Build history of the part. All positions in model axes, mm. Face numbers are marked on the shaded views. A direction names the side the tool comes from. Give positions to 0.01 mm unless a question says otherwise; leave off trailing zeros. Loops run counter-clockwise (first coordinate to the right, second up) from the corner with the lowest first, then second, coordinate; pieces in that order, holes last.
1) Band-saw the part on A-A on z = 4.25. List the corners of the cut face in (x, y), then the cut area to 3 significant figures.
2) Band-saw the part on B-B on y = 15. List the corners of the cut face in (x, z).
3) 3-axis set-ups, long thin cutter, end or side, ignore diameter. For the marked faces 1, 2, 3, 4 and 5: which of +Z, -Z, +X, -X, +Y, -Y reach the whole face in a straight line?
4) Band-saw the part on C-C on x = 18. List the corners of the cut face in (y, z).
5) Wall check: line 1 (X direction, y = 13, z = 7); line 2 (X direction, y = 19.5, z = 3.25); line 3 (Y direction, x = 0.5, z = 9.75). Give the ranges that are in metal, low to high.
6) Two-plate mould, pull along X, no slides. Class the marked faces 6, 7 and 8: +X half, -X half, draft (parallel to the pull), parting line (faces both ways), or undercut.
7) Band-saw the part on D-D on y = 0. List the corners of the cut face in (x, z), then the cut area to 3 significant figures.
8) Flat gauge pins, fed straight in: P1, Ø5.5, axis at y = 21, z = 7.5, coming from the +X side; P2, Ø5, axis at x = 1, z = 3, coming from the +Y side; P3, Ø3, axis at x = 69.5, z = 6.5, coming from the +Y side. Where does each tip first touch, or does it go through?
```python
from build123d import *

# Parameters (mm, degrees)
SKETCH1_R           = 2.5
BOSS_EXTRUDE1_DEPTH = 10


with BuildPart() as part:
    # Sketch1 → Boss-Extrude1 (new body)
    with BuildSketch(Plane.XY):
        with BuildLine():
            Line((-11.526582654, 6), (20.973417346, 6))
            ThreePointArc((20.973417346, 6), (28.044485158, 8.928932188), (30.973417346, 16))
            Line((30.973417346, 16), (30.973417346, 41.837168574))
            ThreePointArc((30.973417346, 41.837168574), (32.455779256, 43.769020227), (34.705468153, 42.837168574))
            Line((34.705468153, 42.837168574), (55.973417346, 6))
            Line((55.973417346, 6), (67.348943548, 12.567663115))
            Line((67.348943548, 12.567663115), (64.080994355, 18.227917153))
            ThreePointArc((64.080994355, 18.227917153), (64.080994355, 20.227917153), (65.813045163, 21.227917153))
            Line((65.813045163, 21.227917153), (72.163898124, 21.227917153))
            ThreePointArc((72.163898124, 21.227917153), (75.663898124, 20.290094979), (78.22607595, 17.727917153))
            Line((78.22607595, 17.727917153), (78.411121374, 17.407409077))
            ThreePointArc((78.411121374, 17.407409077), (79.110424332, 15.719142393), (79.348943548, 13.907409077))
            Line((79.348943548, 13.907409077), (79.348943548, 9.680911769))
            ThreePointArc((79.348943548, 9.680911769), (78.411121374, 6.180911769), (75.848943548, 3.618733942))
            Line((75.848943548, 3.618733942), (60.813163308, -5.062177826))
            ThreePointArc((60.813163308, -5.062177826), (59.124896624, -5.761480784), (57.313163308, -6))
            Line((57.313163308, -6), (-11.526582654, -6))
            ThreePointArc((-11.526582654, -6), (-12.940796217, -5.414213562), (-13.526582654, -4))
            Line((-13.526582654, -4), (-13.526582654, 4))
            ThreePointArc((-13.526582654, 4), (-12.940796217, 5.414213562), (-11.526582654, 6))
        make_face()
        with Locations((-7.526582654, 0)):
            Circle(SKETCH1_R, mode=Mode.SUBTRACT)
        with Locations((7.473417346, 0)):
            Circle(SKETCH1_R, mode=Mode.SUBTRACT)
        with BuildLine():
            Line((50.777264923, 1), (28.973417346, 1))
            ThreePointArc((28.973417346, 1), (35.550797083, 7.253572158), (37.973417346, 16))
            Line((37.973417346, 16), (37.973417346, 23.176914536))
            Line((37.973417346, 23.176914536), (50.777264923, 1))
        make_face(mode=Mode.SUBTRACT)
    extrude(amount=BOSS_EXTRUDE1_DEPTH)


solid = part.part
```
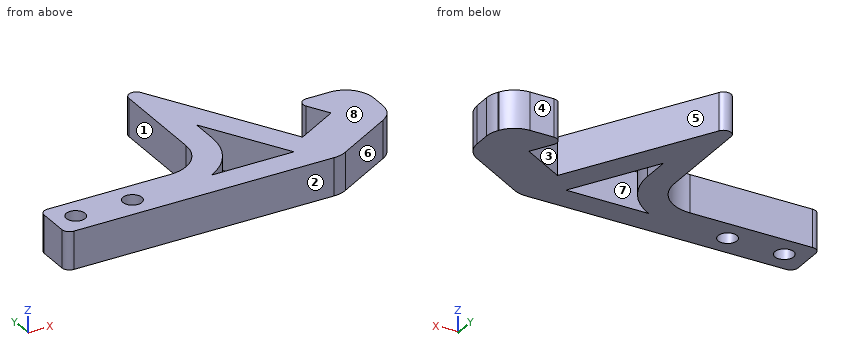
Findings below:
1. outline: (-13.53, -4) arc R2 ccw to (-11.53, -6) - (57.31, -6) arc R7 ccw to (60.81, -5.06) - (75.85, 3.62) arc R7 ccw to (79.35, 9.68) - (79.35, 13.91) arc R7 ccw to (78.41, 17.41) - (78.23, 17.73) arc R7 ccw to (72.16, 21.23) - (65.81, 21.23) arc R2 ccw to (64.08, 18.23) - (67.35, 12.57) - (55.97, 6) - (34.71, 42.84) arc R2 ccw to (30.97, 41.84) - (30.97, 16) arc R10 cw to (20.97, 6) - (-11.53, 6) arc R2 ccw to (-13.53, 4) - close; hole circle Ø5 at (-7.53, 0); hole circle Ø5 at (7.47, 0); hole (28.97, 1) - (50.78, 1) - (37.97, 23.18) - (37.97, 16) arc R17 cw to start
1. area: 1,550 mm2
2. outline: (30.92, 0) - (37.94, 0) - (37.94, 10) - (30.92, 10) - close; (42.69, 0) - (50.78, 0) - (50.78, 10) - (42.69, 10) - close; (65.94, 0) - (79.26, 0) - (79.26, 10) - (65.94, 10) - close
3. face 1: +Z, -Z, -X, +Y
3. face 2: +Z, -Z, +X, -X, -Y
3. face 3: +Z, -Z
3. face 4: +Z, -Z, +X, +Y
3. face 5: +Z, -Z, +Y
4. outline: (-6, 0) - (6, 0) - (6, 10) - (-6, 10) - close
5. line 1: x = 30.51 to 37.71, 43.85 to 51.93, 67.1 to 79.35
5. line 2: x = 30.97 to 37.97, 40.1 to 48.18, 63.83 to 76.77
5. line 3: y = -6 to 6
6. face 6: +X half
6. face 7: undercut
6. face 8: draft
7. outline: (-13.53, 0) - (-10.03, 0) - (-10.03, 10) - (-13.53, 10) - close; (-5.03, 0) - (4.97, 0) - (4.97, 10) - (-5.03, 10) - close; (9.97, 0) - (69.58, 0) - (69.58, 10) - (9.97, 10) - close
7. area: 731 mm2
8. P1: stops at x = 77.89
8. P2: stops at y = 6
8. P3: stops at y = 21.23
